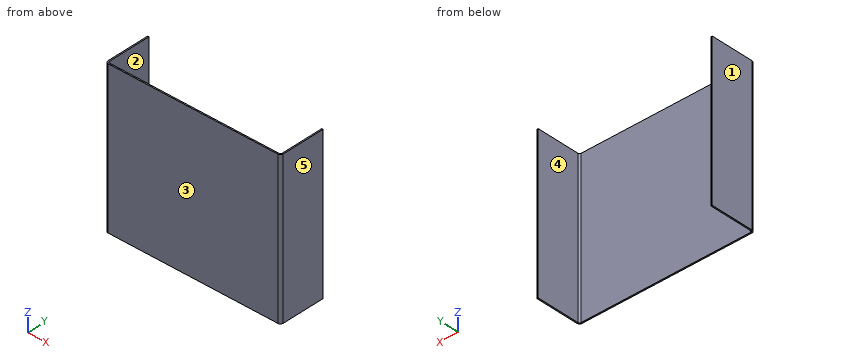
from build123d import *

# Parameters (mm, degrees)
F1_DEPTH = 203.2
F2_R     = 3.69316
F3_R     = 1.98374


with BuildPart() as f1:
    # F0 (on Top) → F1 (new body)
    with BuildSketch(Plane.XY):
        Polygon((0, -59.54209), (0, 0), (-1.70942, 0), (-1.70942, -61.25151), (232.920897, -61.25151), (232.920897, 0), (231.211477, 0), (231.211477, -59.54209), align=None)
    extrude(amount=F1_DEPTH)

    # F2
    f2_edges = [f1.edges().sort_by_distance(p)[0] for p in [
        (232.920897, -61.25151, 101.6),
        (-1.70942, -61.25151, 101.6),
    ]]
    fillet(f2_edges, radius=F2_R)

    # F3
    f3_edges = [f1.edges().sort_by_distance(p)[0] for p in [
        (0, -59.54209, 101.6),
        (231.211477, -59.54209, 101.6),
    ]]
    fillet(f3_edges, radius=F3_R)


solid = f1.part
Geometry: final body of the model. Coordinates: model frame, mm. Face numbers are marked on the shaded views. A direction names the side the tool comes from. Give positions to 0.01 mm unless a question says otherwise; leave off trailing zeros. Loops run counter-clockwise (first coordinate to the right, second up) from the corner with the lowest first, then second, coordinate; pieces in that order, holes last. Notation, with made-up numbers: M 47,-29 L 69,-29 A22 ccw 69,-5 Z; hole C 28.25,-3.5 d3. An arc over 180 degrees is marked long. Put each result on its own line as item: value.
1) Cut plane A-A, the plane y = -26. Return the cut outline in (x, z).
Computed values:
outline: M -1.71,0 L 0,0 L 0,203.2 L -1.71,203.2 Z; M 231.21,0 L 232.92,0 L 232.92,203.2 L 231.21,203.2 Z
2) First-contact query: P1, Ø3, axis at x = 150.5, z = 89.5, coming from the +Y side; P2, Ø10, axis at x = 44.5, y = -50.5, coming from the -Z side. Flat tips, straight axial feed; report the tip coordinate or a pass-through.
Computed values:
P1: stops at y = -59.54
P2: passes through
3) Cut plane B-B, the plane z = 73. Return the cut outline in (x, y).
Computed values:
outline: M -1.71,-57.56 A3.69 ccw 1.98,-61.25 L 229.23,-61.25 A3.69 ccw 232.92,-57.56 L 232.92,0 L 231.21,0 L 231.21,-57.56 A1.98 cw 229.23,-59.54 L 1.98,-59.54 A1.98 cw 0,-57.56 L 0,0 L -1.71,0 Z
4) Material intervals for L1, parallel to X at y = -9, z = 87.5; L2, parallel to Y at x = 207, z = 97.5, sorted ascending. Write a range as from..to.
Computed values:
L1: x = -1.71..0, 231.21..232.92
L2: y = -61.25..-59.54
5) Reachability of the marked faces 4 and 5 from +Z, -Z, +X, -X, +Y, -Y: full face, straight path, thin tool, end or side. Return the list, or none.
Computed values:
face 4: +Z, -Z, +Y
face 5: +Z, -Z, +X, +Y, -Y
6) Cut plane C-C, the plane x = 155.5. Return the cut outline in (y, z).
Computed values:
outline: M -61.25,0 L -59.54,0 L -59.54,203.2 L -61.25,203.2 Z
7) Mould query, pull axis X, two halves, no side actions, for the marked faces 1, 2 and 3. Classes: released by +X, released by -X, zero draft, split by the parting line, or undercut.
Computed values:
face 1: released by -X
face 2: undercut
face 3: zero draft
